Source: CAD feature listing. Evaluate the final solid. Frame: model axes, mm. Face numbers are marked on the shaded views. Round coordinates to 2 decimals unless told otherwise and drop trailing zeros. Write each loop counter-clockwise with the first axis right and the second up, starting at its lowest first coordinate (ties: lowest second). Pieces come first, ordered by that corner, then holes.
from build123d import *

# Parameters (mm, degrees)
F0_W     = 11.58612
F0_H     = 48.573878
F0_R     = 4
F0_R_2   = 3.99
F0_R_3   = 3.98
F0_R_4   = 3.97
F0_R_5   = 3.96
F1_DEPTH = 10
F2_R     = 3.175
F3_DEPTH = 4


with BuildPart() as f1:
    # F0 (on Top) → F1 (new body)
    with BuildSketch(Plane.XY):
        with Locations((5.79306, 24.286939)):
            Rectangle(F0_W, F0_H)
        with Locations((5.79306, 5.655282)):
            Circle(F0_R, mode=Mode.SUBTRACT)
        with Locations((5.79306, 14.755282)):
            Circle(F0_R_2, mode=Mode.SUBTRACT)
        with Locations((5.79306, 23.855282)):
            Circle(F0_R_3, mode=Mode.SUBTRACT)
        with Locations((5.79306, 32.955282)):
            Circle(F0_R_4, mode=Mode.SUBTRACT)
        with Locations((5.79306, 42.055282)):
            Circle(F0_R_5, mode=Mode.SUBTRACT)
    extrude(amount=F1_DEPTH)

    # F2 (on face) → F3 (cut)
    with BuildSketch(Plane.XY.offset(10)):
        with Locations((-0.836659, 0)):
            Circle(F2_R)
    extrude(amount=-F3_DEPTH, mode=Mode.SUBTRACT)


solid = f1.part
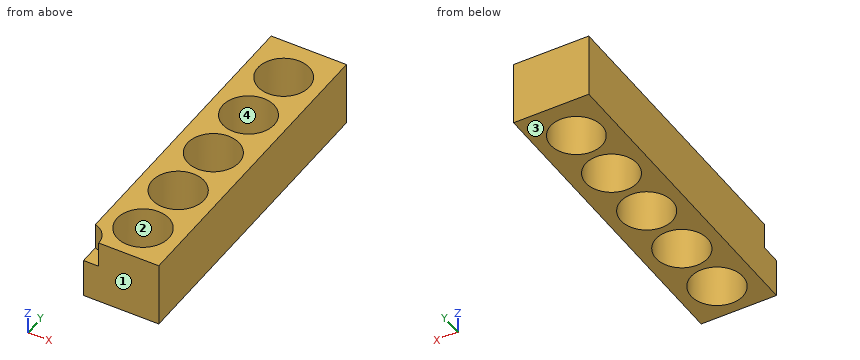
1) Section query D-D on x = 3.75. Return the cut outline in (y, z), then the cut area to 3 significant figures.
Taken from the geometry:
outline: (0, 0) - (2.22, 0) - (2.22, 10) - (0, 10) - close; (9.09, 0) - (11.33, 0) - (11.33, 10) - (9.09, 10) - close; (18.18, 0) - (20.44, 0) - (20.44, 10) - (18.18, 10) - close; (27.27, 0) - (29.55, 0) - (29.55, 10) - (27.27, 10) - close; (36.36, 0) - (38.66, 0) - (38.66, 10) - (36.36, 10) - close; (45.45, 0) - (48.57, 0) - (48.57, 10) - (45.45, 10) - close
area: 144 mm2
2) Section query C-C on z = 2.75. Return the cut outline in (x, y), then the cut area to 3 significant figures.
Taken from the geometry:
outline: (0, 0) - (11.59, 0) - (11.59, 48.57) - (0, 48.57) - close; hole circle Ø8 at (5.79, 5.66); hole circle Ø7.98 at (5.79, 14.76); hole circle Ø7.96 at (5.79, 23.86); hole circle Ø7.94 at (5.79, 32.96); hole circle Ø7.92 at (5.79, 42.06)
area: 314 mm2
3) Section query A-A on x = 8.25. Return the cut outline in (y, z), then the cut area to 3 significant figures.
Taken from the geometry:
outline: (0, 0) - (2.5, 0) - (2.5, 10) - (0, 10) - close; (8.81, 0) - (11.61, 0) - (11.61, 10) - (8.81, 10) - close; (17.9, 0) - (20.72, 0) - (20.72, 10) - (17.9, 10) - close; (26.99, 0) - (29.84, 0) - (29.84, 10) - (26.99, 10) - close; (36.07, 0) - (38.95, 0) - (38.95, 10) - (36.07, 10) - close; (45.16, 0) - (48.57, 0) - (48.57, 10) - (45.16, 10) - close
area: 173 mm2
4) Material intervals for line 1 (Y direction, x = 5.5, z = 6); line 2 (X direction, y = 23.5, z = 3.5); line 3 (Y direction, x = 8, z = 4.5), sorted ascending.
Taken from the geometry:
line 1: y = 0 to 1.67, 9.64 to 10.78, 18.73 to 19.89, 27.82 to 29, 36.91 to 38.11, 46 to 48.57
line 2: x = 0 to 1.83, 9.76 to 11.59
line 3: y = 0 to 2.32, 8.99 to 11.43, 18.08 to 20.54, 27.17 to 29.66, 36.26 to 38.77, 45.34 to 48.57
5) Pull-direction query (Y, two-part tool) for the marked faces 1, 2, 3 and 4; classes: released by +Y, released by -Y, zero draft, split by the parting line, or undercut.
Taken from the geometry:
face 1: released by -Y
face 2: undercut
face 3: zero draft
face 4: undercut
6) Section query B-B on y = 39. Return the cut outline in (x, z).
Taken from the geometry:
outline: (0, 0) - (3.27, 0) - (3.27, 10) - (0, 10) - close; (8.31, 0) - (11.59, 0) - (11.59, 10) - (8.31, 10) - close
